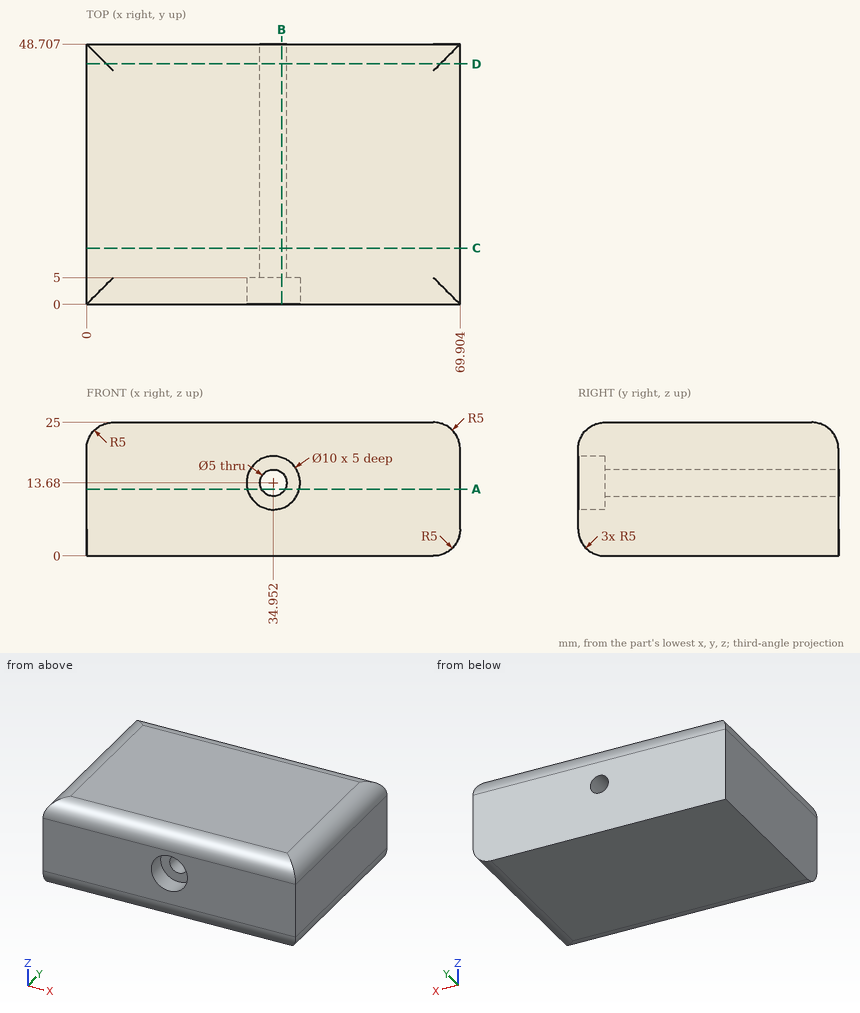
For this review, use the dimensioned drawing (mm, ordinates from the lowest corner) and the shaded views. Round coordinates to 2 decimals unless told otherwise and drop trailing zeros. Order: outer loops, then holes, each group sorted by start corner. A loop starts at its lowest first (then second) coordinate and runs counter-clockwise, first axis right, second up.
1) Clearance check with flat-ended pins moving along their axes: pin 1 Ø4.5 at (x, z) = (34.95, 13.68) entering from +Y; pin 2 Ø3 at (x, z) = (37.5, 15.5) entering from -Y. State where each tip first meets the part, or that it passes through.
The answers:
pin 1: passes through
pin 2: stops at y = 5
2) Consider section D-D (y = 45). State the section outline as (x, z) points (1 decimal), plus the area to 3 significant figures.
The answers:
outline: (0, 0) - (64.9, 0) arc R5 ccw to (69.9, 5) - (69.9, 20) arc R5 ccw to (66.2, 24.8) - (3.7, 24.8) arc R5 ccw to (0, 20) - close; hole circle Ø5 at (35, 13.7)
area: 1,700 mm2
3) Consider section B-B (x = 36.5). State the section outline as (y, z) points (1 decimal).
The answers:
outline: (0, 5) arc R5 ccw to (5, 0) - (48.7, 0) - (48.7, 11.7) - (5, 11.7) - (5, 8.9) - (0, 8.9) - close; (0, 18.4) - (5, 18.4) - (5, 15.6) - (48.7, 15.6) - (48.7, 20) arc R5 ccw to (43.7, 25) - (5, 25) arc R5 ccw to (0, 20) - close
4) Consider section C-C (y = 10.5). State the section outline as (x, z) points (1 decimal).
The answers:
outline: (0, 0) - (64.9, 0) arc R5 ccw to (69.9, 5) - (69.9, 20) arc R5 ccw to (64.9, 25) - (5, 25) arc R5 ccw to (0, 20) - close; hole circle Ø5 at (35, 13.7)
5) Consider section A-A (z = 12.5). State the section outline as (x, y) points (1 decimal), plus the area to 3 significant figures.
The answers:
outline: (0, 0) - (30.1, 0) - (30.1, 5) - (32.7, 5) - (32.7, 48.7) - (0, 48.7) - close; (37.2, 5) - (39.8, 5) - (39.8, 0) - (69.9, 0) - (69.9, 48.7) - (37.2, 48.7) - close
area: 3,160 mm2
6) For L1, parallel to Z at x = 36.5, y = 34.5 (1 decimal); L2, parallel to Y at x = 11.5, z = 4.5 (1 decimal); L3, parallel to Y at x = 61, z = 1 (1 decimal), list the stretches that pass through material, from the lowest coordinate up.
The answers:
L1: z = 0 to 11.7, 15.6 to 25
L2: y = 0 to 48.7
L3: y = 2 to 48.7
